```python
from build123d import *

# Parameters (mm, degrees)
ESQUISSE_CORPS_R   = 34.9
BOSS_EXTRU_1_DEPTH = 3
ESQUISSE5_R        = 1.5
BOSS_EXTRU_2_DEPTH = 3
ESQUISSE6_R        = 1.15
BOSS_EXTRU_3_DEPTH = 2
ESQUISSE7_R        = 34.9
ESQUISSE7_R_2      = 32.9
BOSS_EXTRU_4_DEPTH = 9


with BuildPart() as part:
    # Esquisse_corps → Boss.-Extru.1 (new body)
    with BuildSketch(Plane.XY):
        Circle(ESQUISSE_CORPS_R)
        with BuildLine():
            ThreePointArc((-11.220011679, -26.953884347), (-7.983884347, -25.529988321), (-6.559988321, -28.766115653))
            ThreePointArc((-6.559988321, -28.766115653), (-6.289235285, -31.30799577), (-4.108913196, -32.642408495))
            ThreePointArc((-4.108913196, -32.642408495), (0, -32.9), (4.108913196, -32.642408495))
            ThreePointArc((4.108913196, -32.642408495), (6.289235285, -31.30799577), (6.559988321, -28.766115653))
            ThreePointArc((6.559988321, -28.766115653), (7.983884347, -25.529988321), (11.220011679, -26.953884347))
            ThreePointArc((11.220011679, -26.953884347), (13.316969942, -28.87783046), (16.154521733, -28.660799493))
            ThreePointArc((16.154521733, -28.660799493), (32.305537105, -6.225935459), (25.64893396, 20.604421533))
            ThreePointArc((25.64893396, 20.604421533), (17.65423242, 21.86309032), (11.220011679, 16.953884347))
            ThreePointArc((11.220011679, 16.953884347), (7.983884347, 15.529988321), (6.559988321, 18.766115653))
            ThreePointArc((6.559988321, 18.766115653), (6.487068724, 27.321563828), (0, 32.9))
            ThreePointArc((0, 32.9), (-6.487068724, 27.321563828), (-6.559988321, 18.766115653))
            ThreePointArc((-6.559988321, 18.766115653), (-7.983884347, 15.529988321), (-11.220011679, 16.953884347))
            ThreePointArc((-11.220011679, 16.953884347), (-17.65423242, 21.86309032), (-25.64893396, 20.604421533))
            ThreePointArc((-25.64893396, 20.604421533), (-32.305537105, -6.225935459), (-16.154521733, -28.660799493))
            ThreePointArc((-16.154521733, -28.660799493), (-13.316969942, -28.87783046), (-11.220011679, -26.953884347))
        make_face(mode=Mode.SUBTRACT)
    extrude(amount=BOSS_EXTRU_1_DEPTH)

    # Esquisse5 → Boss.-Extru.2 (add)
    with BuildSketch(Plane.XY.offset(3)):
        with Locations((-8.89, 17.86)):
            Circle(ESQUISSE5_R)
        with Locations((-8.89, -27.86)):
            Circle(ESQUISSE5_R)
        with Locations(Location((8.89, -27.86, 0), (0, 0, 180))):
            Circle(ESQUISSE5_R)
        with Locations(Location((8.89, 17.86, 0), (0, 0, 180))):
            Circle(ESQUISSE5_R)
    extrude(amount=BOSS_EXTRU_2_DEPTH)

    # Esquisse6 → Boss.-Extru.3 (add)
    with BuildSketch(Plane.XY.offset(6)):
        with Locations((-8.89, 17.86)):
            Circle(ESQUISSE6_R)
        with Locations((-8.89, -27.86)):
            Circle(ESQUISSE6_R)
        with Locations(Location((8.89, -27.86, 0), (0, 0, 180))):
            Circle(ESQUISSE6_R)
        with Locations(Location((8.89, 17.86, 0), (0, 0, 180))):
            Circle(ESQUISSE6_R)
    extrude(amount=BOSS_EXTRU_3_DEPTH)

    # Esquisse7 → Boss.-Extru.4 (add)
    with BuildSketch(Plane.XY.offset(3)):
        Circle(ESQUISSE7_R)
        with Locations(Location((0, 0, 0), (0, 0, 141.224227635))):
            Circle(ESQUISSE7_R_2, mode=Mode.SUBTRACT)
    extrude(amount=BOSS_EXTRU_4_DEPTH)


solid = part.part
```
The model under review builds one solid part; all positions refer to its coordinate system, in mm. A direction names the side the tool comes from. Round coordinates to 2 decimals unless told otherwise and drop trailing zeros. Loops run counter-clockwise (first coordinate to the right, second up) from the corner with the lowest first, then second, coordinate; pieces in that order, holes last. Notation, with made-up numbers: (72.25, 66) -> (79.25, 66) arc R17 cw to (79.25, 75) -> close; hole circle Ø5 at (15.25, -8). An arc over 180 degrees is marked (long way). Answer in a Markdown table with one row per item.
1) Wall thickness on line 1 along Y through (x, z) = (0, 8.5); line 2 along Z through (x, y) = (-10, -27); line 3 along X through (y, z) = (-3, 9): over which ranges is each line inside the solid? List them lowest first.
Taken from the geometry:
| item | result |
|---|---|
| line 1 | y = -34.9 to -32.9, 32.9 to 34.9 |
| line 2 | z = 0 to 6 |
| line 3 | x = -34.77 to -32.76, 32.76 to 34.77 |
2) Consider section A-A, the plane z = 4.5. Write out the cut boundary in (x, y), plus the area to 3 significant figures.
Taken from the geometry:
| item | result |
|---|---|
| outline | circle Ø69.8 at (0, 0); circle Ø3 at (-8.89, -27.86); circle Ø3 at (-8.89, 17.86); circle Ø3 at (8.89, -27.86); circle Ø3 at (8.89, 17.86); hole circle Ø65.8 at (0, 0) |
| area | 454 mm² |
3) For pin 1 Ø8 at (x, y) = (-14, -19.5) entering from -Z; pin 2 Ø1.5 at (y, z) = (-11, 9.5) entering from +X; pin 3 Ø1.5 at (x, y) = (-9.5, 18.5) entering from +Z; pin 4 Ø9 at (x, y) = (9.5, 25.5) entering from +Z, all flat-tipped, find the tip position at first contact; note any pin that passes through.
Taken from the geometry:
| item | result |
|---|---|
| pin 1 | passes through |
| pin 2 | stops at x = 33.36 |
| pin 3 | stops at z = 8 |
| pin 4 | stops at z = 3 |
4) Tool access review of faces 1 (the flat face through (9, 18, 8)), 2 (the cylindrical face through (-17.542, 21.834, 1.479)): name each direction out of +Z, -Z, +X, -X, +Y, -Y from which nothing blocks a thin tool from reaching the whole face with its end or side.
Taken from the geometry:
| item | result |
|---|---|
| face 1 | +Z |
| face 2 | +Z, -Z |
5) Consider section B-B, the plane y = 0. Write out the cut boundary in (x, z), plus the area to 3 significant figures.
Taken from the geometry:
| item | result |
|---|---|
| outline | (-34.9, 0) -> (-32.9, 0) -> (-32.9, 12) -> (-34.9, 12) -> close; (32.9, 0) -> (34.9, 0) -> (34.9, 12) -> (32.9, 12) -> close |
| area | 48.0 mm² |
6) Consider section C-C, the plane x = 15. Write out the cut boundary in (y, z), plus the area to 3 significant figures.
Taken from the geometry:
| item | result |
|---|---|
| outline | (-31.51, 0) -> (-29.04, 0) -> (-29.04, 3) -> (-29.28, 3) -> (-29.28, 12) -> (-31.51, 12) -> close; (20.78, 0) -> (31.51, 0) -> (31.51, 12) -> (29.28, 12) -> (29.28, 3) -> (20.78, 3) -> close |
| area | 79.8 mm² |
7) Draft analysis for pull direction X (two halves, no side actions). For faces 3 (the flat face through (13, 24, 3)), 4 (the flat face through (-8, 16, 0)), 5 (the cylindrical face through (-7.57, -34.07, 5.92)), state which applies: pulls with the +X half, pulls with the -X half, needs draft (parallel to the pull), parting line crosses it, or undercut.
Taken from the geometry:
| item | result |
|---|---|
| face 3 | undercut |
| face 4 | needs draft |
| face 5 | parting line crosses it |
8) Consider section D-D, the plane y = -27.86. Count the separate pieces of the cut face and the enclosed holes in it, plus the area to 3 significant figures.
Taken from the geometry:
| item | result |
|---|---|
| separate pieces | 4 |
| enclosed holes | 0 |
| area | 144 mm² |
